```python
from build123d import *

# Parameters (mm, degrees)
BOSS_EXTRUDE1_DEPTH = 1.5
SKETCH2_R           = 1.6
CUT_EXTRUDE1_DEPTH  = 3.5


with BuildPart() as part:
    # Sketch1 → Boss-Extrude1 (new body)
    with BuildSketch(Plane.XY):
        Polygon((-586.414001465, 117.914742868), (-828.47776474, 117.914742868), (-828.47776474, -10.5), (-586.414001465, -10.5), (-578.414001465, -2.5), (-578.414001465, 109.914742868), align=None)
        Polygon((-613.414001465, 4.5), (-600.414001465, 4.5), (-590.414001465, 14.5), (-590.414001465, 92.914742868), (-600.414001465, 102.914742868), (-613.414001465, 102.914742868), align=None, mode=Mode.SUBTRACT)
    extrude(amount=BOSS_EXTRUDE1_DEPTH)

    # Sketch2 → Cut-Extrude1 (cut)
    with BuildSketch(Plane.XY.offset(1.5)):
        with Locations((-818.47776474, -4.5)):
            Circle(SKETCH2_R)
        with Locations((-800.992483366, -4.5)):
            Circle(SKETCH2_R)
        with Locations((-623.414001465, -4.5)):
            Circle(SKETCH2_R)
        with Locations((-588.414001465, -4.5)):
            Circle(SKETCH2_R)
        with Locations((-623.414001465, 111.914742868)):
            Circle(SKETCH2_R)
        with Locations((-588.414001465, 111.914742868)):
            Circle(SKETCH2_R)
        with Locations((-818.47776474, 111.914742868)):
            Circle(SKETCH2_R)
        with Locations((-800.992483366, 111.914742868)):
            Circle(SKETCH2_R)
    extrude(amount=-CUT_EXTRUDE1_DEPTH, mode=Mode.SUBTRACT)


solid = part.part
```
Part model, mm, in its own coordinate system. A direction names the side the tool comes from. Round coordinates to 2 decimals unless told otherwise and drop trailing zeros. Write each loop counter-clockwise with the first axis right and the second up, starting at its lowest first coordinate (ties: lowest second). Pieces come first, ordered by that corner, then holes. Notation, with made-up numbers: M 10.25,-1.5 L 15.25,-1.5 A24 cw 15.25,28.5 Z; hole C 69.5,87.5 d10. An arc over 180 degrees is marked long. Answer as CSV lines item,"result". Start each with the question number.
1) Drill centre lines: L1, parallel to X at y = 40, z = 0.1; L2, parallel to Y at x = -589, z = 1.05; L3, parallel to X at y = -5, z = 0.1. Where is each one in solid material? Low to high.
2) Band-saw the part on A-A (y = 63). List the corners of the cut face in (x, z).
3) Drop flat-ended pins along their axis: pin 1 (3.5 mm diameter, centred on x = -623.41, y = -4.5, fed in from +Z); pin 2 (3 mm diameter, centred on x = -800.99, y = -4.5, fed in from +Z). Give the stop position or say it passes through.
4) Band-saw the part on B-B (z = 0.3). Count the separate pieces of the cut face and the enclosed holes in it, then the cut area to 3 significant figures.
5) Mould opens along X. For faces 1 (the face through (-582.4, 113.9, 0.7)), 2 (the face through (-705, 55, 0)), 3 (the face through (-595.484, 9.43, 0.74)) say: +X half, -X half, draft (parallel to the pull), parting line (faces both ways), or undercut.
6) Which spindle directions (+Z, -Z, +X, -X, +Y, -Y) get a long thin tool onto all of the face, cutting with end or side? Do faces 4 (the face through (-705, 55, 1.5)), 5 (the face through (-595.3, 97.8, 0.7)). Say none if no direction does.
7) Band-saw the part on C-C (y = 7). List the corners of the cut face in (x, z), then the cut area to 3 significant figures.
Worked out:
1,L1,"-828.48 to -613.41, -590.41 to -578.41"
1,L2,"-10.5 to -5.99, -3.01 to 110.43, 113.4 to 117.91"
1,L3,"-828.48 to -820, -816.96 to -802.51, -799.47 to -624.93, -621.89 to -589.93, -586.89 to -580.91"
2,outline,"M -828.48,0 L -613.41,0 L -613.41,1.5 L -828.48,1.5 Z; M -590.41,0 L -578.41,0 L -578.41,1.5 L -590.41,1.5 Z"
3,pin 1,"z = 1.5"
3,pin 2,"through"
4,separate pieces,"1"
4,enclosed holes,"9"
4,area,"29,800 mm²"
5,face 1,"+X half"
5,face 2,"draft"
5,face 3,"undercut"
6,face 4,"+Z, +X, -X, +Y, -Y"
6,face 5,"+Z, -Z"
7,outline,"M -828.48,0 L -613.41,0 L -613.41,1.5 L -828.48,1.5 Z; M -597.91,0 L -578.41,0 L -578.41,1.5 L -597.91,1.5 Z"
7,area,"352 mm²"
